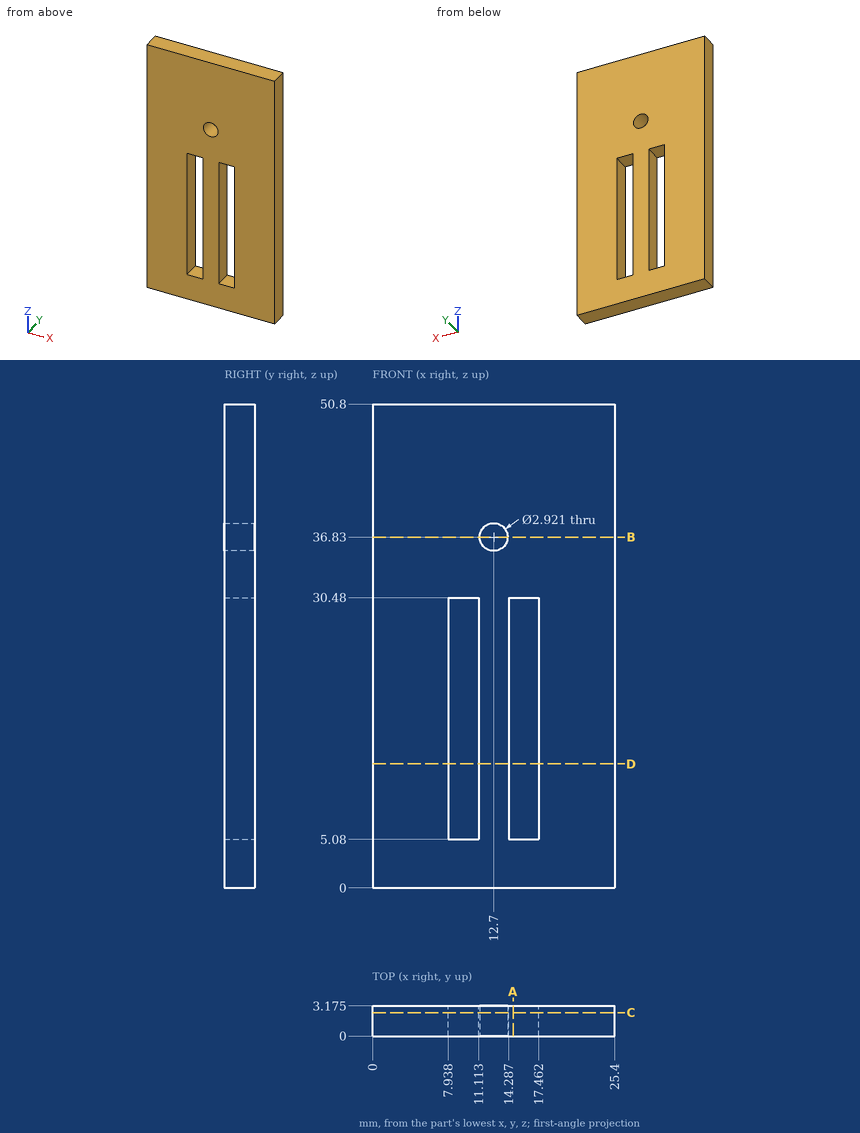
Could you check a few things on this drawing? It's one solid part, dimensions in mm from its lowest x, y, z. Coordinates: 2 decimals unless noted, no trailing zeros. Order: outer loops, then holes, each group sorted by start corner. A loop starts at its lowest first (then second) coordinate and runs counter-clockwise, first axis right, second up. Notation, with made-up numbers: (56.5, 79) - (100.5, 79) arc R13 ccw to (100.5, 85) - close; hole circle Ø2 at (-25, 83.25). An arc over 180 degrees is marked (long way). One line per question, with ' | ' between items.
(1) If I drill on L1, parallel to X at y = 0.2, z = 13.5; L2, parallel to X at y = 2.1, z = 36.83; L3, parallel to Z at x = 16.75, y = 1.7, over which ranges is the centre line in solid material (lowest first)?
Report:
L1: x = 0 to 7.94, 11.11 to 14.29, 17.46 to 25.4 | L2: x = 0 to 11.24, 14.16 to 25.4 | L3: z = 0 to 5.08, 30.48 to 50.8
(2) Suppose I cut it at D-D on z = 13. List the corners of the cut face in (x, y) for me (1 decimal).
Report:
outline: (0, 0) - (7.9, 0) - (7.9, 3.2) - (0, 3.2) - close; (11.1, 0) - (14.3, 0) - (14.3, 3.2) - (11.1, 3.2) - close; (17.5, 0) - (25.4, 0) - (25.4, 3.2) - (17.5, 3.2) - close
(3) Suppose I cut it at A-A on x = 14.75. List the corners of the cut face in (y, z) for me (1 decimal).
Report:
outline: (0, 0) - (3.2, 0) - (3.2, 5.1) - (0, 5.1) - close; (0, 30.5) - (3.2, 30.5) - (3.2, 50.8) - (0, 50.8) - close
(4) Suppose I cut it at B-B on z = 36.83. List the corners of the cut face in (x, y) for me (1 decimal).
Report:
outline: (0, 0) - (11.2, 0) - (11.2, 3.2) - (0, 3.2) - close; (14.2, 0) - (25.4, 0) - (25.4, 3.2) - (14.2, 3.2) - close
(5) Suppose I cut it at C-C on y = 2.45. List the corners of the cut face in (x, z) for me.
Report:
outline: (0, 0) - (25.4, 0) - (25.4, 50.8) - (0, 50.8) - close; hole (7.94, 5.08) - (11.11, 5.08) - (11.11, 30.48) - (7.94, 30.48) - close; hole circle Ø2.92 at (12.7, 36.83); hole (14.29, 5.08) - (17.46, 5.08) - (17.46, 30.48) - (14.29, 30.48) - close
